Could you check a few things on this drawing? It's one solid part, dimensions in mm from its lowest x, y, z. A direction names the side the tool comes from. Round coordinates to 2 decimals unless told otherwise and drop trailing zeros. Return JSON: item names as keys, results as strings.
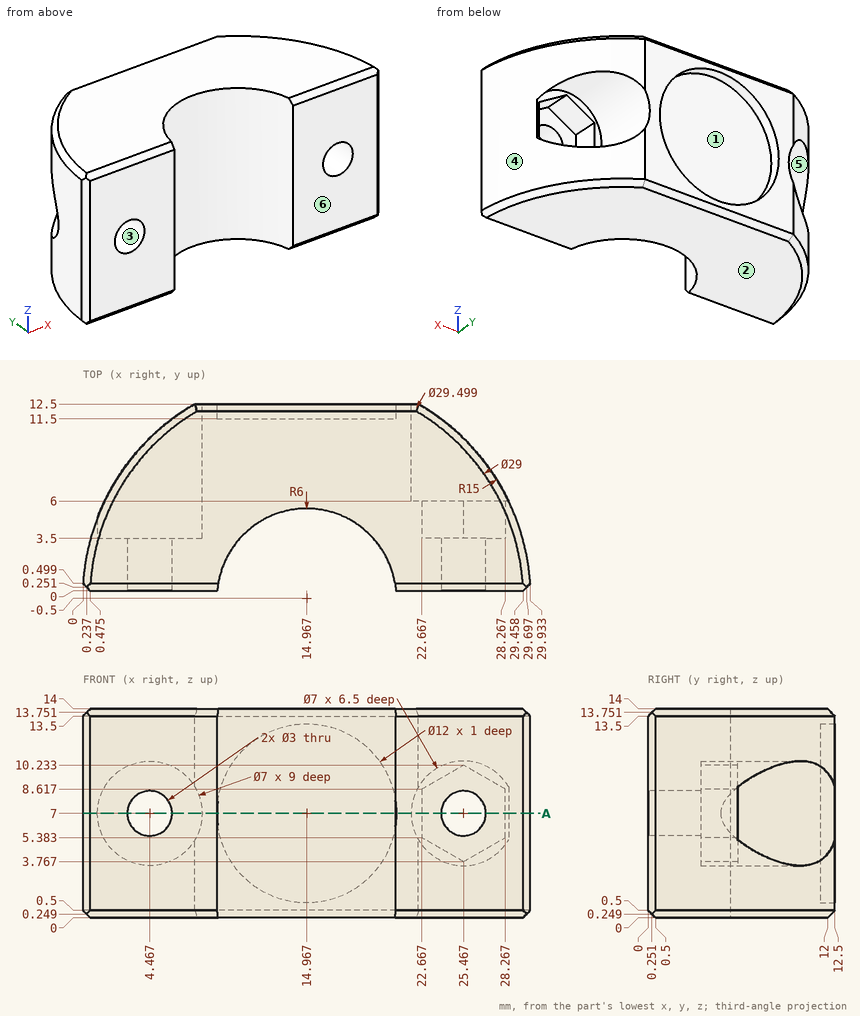
Q1. Suppose I cut it at A-A, the plane z = 7. State how many separate pieces and enclosed holes the cut face has, plus the area to 3 significant figures.
Results:
{"separate pieces": "3", "enclosed holes": "0", "area": "150 mm2"}
Q2. If I drill on line 1 along X through (y, z) = (12, 7); line 2 along Y through (x, z) = (10.75, 12.75); line 3 along Y through (x, z) = (25, 9), over which ranges is the centre line in solid material (lowest first)?
Results:
{"line 1": "x = 7.97 to 8.97, 20.97 to 21.97", "line 2": "y = 3.77 to 12.5", "line 3": "y = 0 to 3.5"}
Q3. Thinking about a two-plate mould opening in X: for the marked faces 3, 4, 5 and 6, which applies, pulls with the +X half, pulls with the -X half, needs draft (parallel to the pull), parting line crosses it, or undercut?
Results:
{"face 3": "undercut", "face 4": "pulls with the +X half", "face 5": "undercut", "face 6": "needs draft"}
Q4. I'm going to push flat-ended pins straight in: pin 1 Ø5.5 at (x, z) = (4.47, 7) entering from +Y; pin 2 Ø1.2 at (y, z) = (5, 7.5) entering from +X; pin 3 Ø0.8 at (y, z) = (5, 7) entering from -X. Where does each tip first touch, or does it pass through?
Results:
{"pin 1": "stops at y = 3.5", "pin 2": "stops at x = 29.14", "pin 3": "stops at x = 0.86"}
Q5. On a 3-axis mill with a long thin cutter (end or side, diameter ignored), from which of +Z, -Z, +X, -X, +Y, -Y can I reach the whole of each face in a straight line? I mean the marked faces 1 and 2. Say none if no direction works.
Results:
{"face 1": "+Y", "face 2": "-Z, +X, -X, +Y, -Y"}
